Geometry: see drawing. Coordinates: mm, zero at the bounding-box minimum. A direction names the side the tool comes from. Give positions to 0.01 mm unless a question says otherwise; leave off trailing zeros. Order: outer loops, then holes, each group sorted by start corner. A loop starts at its lowest first (then second) coordinate and runs counter-clockwise, first axis right, second up. Notation, with made-up numbers: (42, 69) - (86, 69) arc R21 cw to (86, 99) - close; hole circle Ø2 at (-23.75, -2.5). An arc over 180 degrees is marked (long way). One line per item, written item: value.
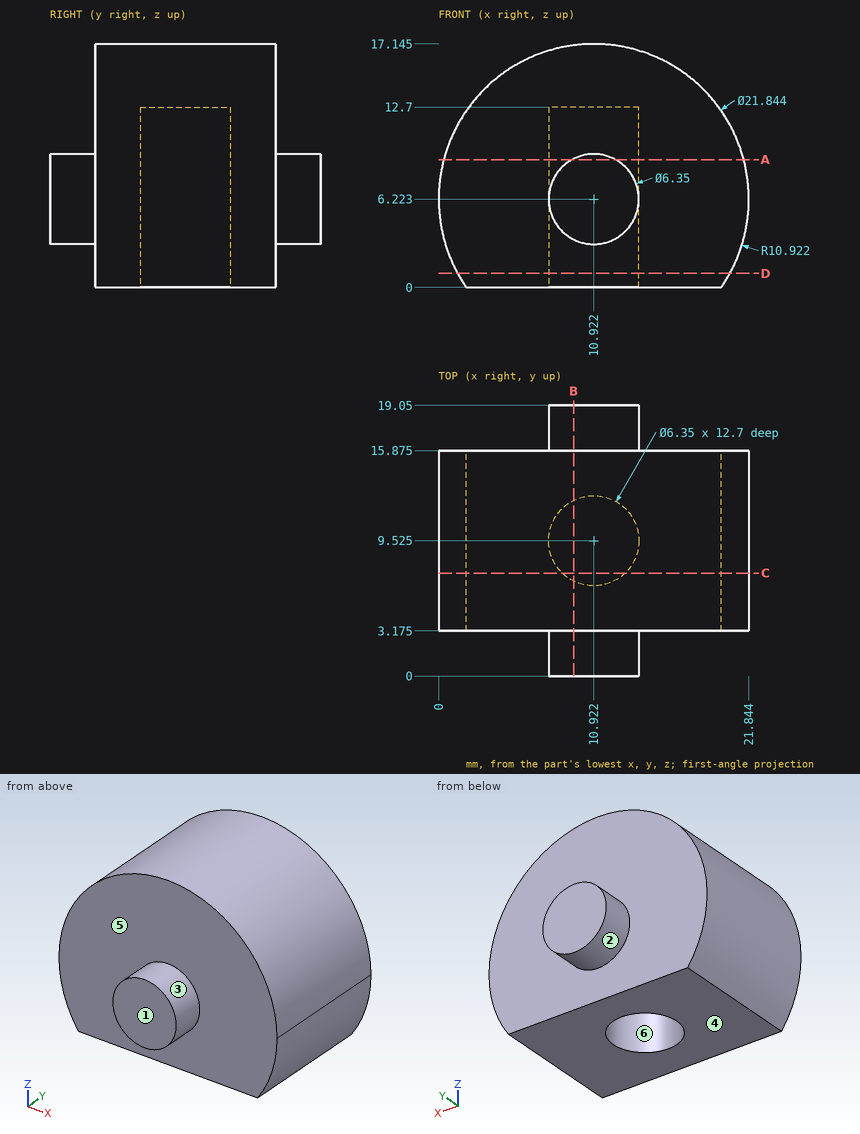
1) Mould query, pull axis Y, two halves, no side actions, for the marked faces 4, 5 and 6. Classes: released by +Y, released by -Y, zero draft, split by the parting line, or undercut.
Answers below:
face 4: zero draft
face 5: released by -Y
face 6: undercut
2) Section C-C, the plane y = 7.25. Return loops of the section in (x, z).
Answers below:
outline: (1.95, 0) - (8.71, 0) - (8.71, 12.7) - (13.14, 12.7) - (13.14, 0) - (19.9, 0) arc R10.92 ccw to (21.84, 6.22) arc R10.92 ccw (long way) to start
3) Section B-B, the plane x = 9.5. Return loops of the section in (y, z) (3 decimals), then the cut area to 3 significant figures.
Answers below:
outline: (0, 3.384) - (3.175, 3.384) - (3.175, 0) - (6.686, 0) - (6.686, 12.7) - (12.364, 12.7) - (12.364, 0) - (15.875, 0) - (15.875, 3.384) - (19.05, 3.384) - (19.05, 9.062) - (15.875, 9.062) - (15.875, 17.052) - (3.175, 17.052) - (3.175, 9.062) - (0, 9.062) - close
area: 181 mm^2
4) Material intervals for line 1 along Y through (x, z) = (15.75, 10.75) (3 decimals); line 2 along X through (y, z) = (12, 6.5); line 3 along X through (y, z) = (7.25, 10.25), sorted ascending.
Answers below:
line 1: 3.175 to 15.875
line 2: 0 to 8.93, 12.91 to 21.84
line 3: 0.77 to 8.71, 13.14 to 21.07
5) Set-up query: the marked faces 1, 2 and 3. Return all of +Z, -Z, +X, -X, +Y, -Y with unobstructed straight access to the full face (end or side cutting, diameter ignored); none if empty.
Answers below:
face 1: +Z, -Z, +X, -X, -Y
face 2: +Y
face 3: -Y
6) First-contact query: pin 1 (8 mm diameter, centred on x = 9, z = 4, fed in from -Y); pin 2 (1 mm diameter, centred on x = 14, z = 11.5, fed in from -Y) (3 decimals); pin 3 (4 mm diameter, centred on x = 7, z = 14.5, fed in from +Y) (3 decimals); pin 4 (2 mm diameter, centred on x = 14, y = 8, fed in from +Z). Flat tips, straight axial feed; report the tip coordinate or a pass-through.
Answers below:
pin 1: y = 0
pin 2: y = 3.175
pin 3: y = 15.875
pin 4: z = 16.95
7) Section A-A, the plane z = 9. Return loops of the section in (x, y) (3 decimals), then the cut area to 3 significant figures.
Answers below:
outline: (0.359, 3.175) - (9.383, 3.175) - (9.383, 0) - (12.461, 0) - (12.461, 3.175) - (21.485, 3.175) - (21.485, 15.875) - (12.461, 15.875) - (12.461, 19.05) - (9.383, 19.05) - (9.383, 15.875) - (0.359, 15.875) - close; hole circle Ø6.35 at (10.922, 9.525)
area: 256 mm^2
8) Section D-D, the plane z = 1. Return loops of the section in (x, y) (3 decimals).
Answers below:
outline: (1.33, 3.175) - (20.514, 3.175) - (20.514, 15.875) - (1.33, 15.875) - close; hole circle Ø6.35 at (10.922, 9.525)
